Could you check a few things on this model? Use its own coordinates, in mm. A direction names the side the tool comes from. Round coordinates to 2 decimals unless told otherwise and drop trailing zeros. Order: outer loops, then holes, each group sorted by start corner. A loop starts at its lowest first (then second) coordinate and runs counter-clockwise, first axis right, second up. Notation, with made-up numbers: M 5,62.25 L 15,62.25 A21 cw 15,93.25 Z; hole C 50.5,70 d8. An arc over 180 degrees is marked long. Write each question's results on one line, items separated by ' | '. Start each with the question number.
1. Suppose I cut it at D-D on x = -0.4. Write out the boundary of the cut face in (y, z).
2. I'm going to push flat-ended pins straight in: pin 1 (1 mm diameter, centred on y = 1.5, z = -1.5, fed in from -X); pin 2 (1.5 mm diameter, centred on y = -0.5, z = -1.5, fed in from +X); pin 3 (0.8 mm diameter, centred on y = 0, z = -3, fed in from -X); pin 4 (1 mm diameter, centred on x = 0.5, y = 1.5, fed in from -Z). Where does each tip first touch, or does it pass through?
3. Suppose I cut it at C-C on z = -0.5. Write out the boundary of the cut face in (x, y).
4. Suppose I cut it at B-B on x = 1.35. Write out the boundary of the cut face in (y, z).
5. Please list where these lines run through material, in increasing order: L1, parallel to X at y = -1.2, z = -2.5; L2, parallel to Z at x = -0.4, y = 0.55; L3, parallel to Z at x = 1.5, y = -0.25.
6. For faces 1 (the flat face through (1.05, 0, -2)), 2 (the flat face through (1.55, 0, -2)), 3 (the flat face through (1.75, 0, 1)), which set-ups out of +Z, -Z, +X, -X, +Y, -Y let a thin tool reach every point of the face, with its end or its side?
7. Suppose I cut it at A-A on y = 0. Write out the boundary of the cut face in (x, z).
from build123d import *

# Parameters (mm, degrees)
SKETCH1_W           = 3.5
SKETCH1_H           = 6
BOSS_EXTRUDE1_DEPTH = 2
SKETCH2_W           = 0.5
SKETCH2_H           = 2.5
BOSS_EXTRUDE2_DEPTH = 5
FILLET1_R           = 1
CUT_EXTRUDE1_DEPTH  = 5


with BuildPart() as part:
    # Sketch1 → Boss-Extrude1 (new body)
    with BuildSketch(Plane.XY):
        Rectangle(SKETCH1_W, SKETCH1_H)
    extrude(amount=BOSS_EXTRUDE1_DEPTH)

    # Sketch2 → Boss-Extrude2 (add)
    with BuildSketch(Plane(origin=(0, 0, 0), x_dir=(-1, 0, 0), z_dir=(0, 0, -1))):
        with Locations((-1.3, 0)):
            Rectangle(SKETCH2_W, SKETCH2_H)
    extrude(amount=BOSS_EXTRUDE2_DEPTH)

    # Fillet1
    fillet1_edges = [part.edges().sort_by_distance(p)[0] for p in [
        (1.3, 1.25, -5),
        (1.3, -1.25, -5),
    ]]
    fillet(fillet1_edges, radius=FILLET1_R)

    # Sketch3 → Cut-Extrude1 (cut)
    with BuildSketch(Plane(origin=(1.55, 0, 0), x_dir=(0, 0, -1), z_dir=(1, 0, 0))):
        with BuildLine():
            Line((2.7, 0.5), (3.7, 0.5))
            ThreePointArc((3.7, 0.5), (4.2, 0), (3.7, -0.5))
            Line((3.7, -0.5), (2.7, -0.5))
            ThreePointArc((2.7, -0.5), (2.2, 0), (2.7, 0.5))
        make_face()
    extrude(amount=-CUT_EXTRUDE1_DEPTH, mode=Mode.SUBTRACT)


solid = part.part
Filled sheet:
1) outline: M -3,0 L 3,0 L 3,2 L -3,2 Z
2) pin 1: stops at x = 1.05 | pin 2: stops at x = 1.55 | pin 3: passes through | pin 4: stops at z = 0
3) outline: M 1.05,-1.25 L 1.55,-1.25 L 1.55,1.25 L 1.05,1.25 Z
4) outline: M -3,0 L -1.25,0 L -1.25,-4 A1 ccw -0.25,-5 L 0.25,-5 A1 ccw 1.25,-4 L 1.25,0 L 3,0 L 3,2 L -3,2 Z; hole M -0.5,-3.7 A0.5 ccw 0.5,-3.7 L 0.5,-2.7 A0.5 ccw -0.5,-2.7 Z
5) L1: x = 1.05 to 1.55 | L2: z = 0 to 2 | L3: z = -5 to -4.13, -2.27 to 2
6) face 1: -Z, -X, +Y, -Y | face 2: -Z, +X, +Y, -Y | face 3: +Z, -Z, +X, +Y, -Y
7) outline: M -1.75,0 L 1.05,0 L 1.05,-2.2 L 1.55,-2.2 L 1.55,0 L 1.75,0 L 1.75,2 L -1.75,2 Z; M 1.05,-5 L 1.55,-5 L 1.55,-4.2 L 1.05,-4.2 Z
